```python
from build123d import *

# Parameters (mm, degrees)
SKETCH_W           = 2
SKETCH_H           = 70
PAD_DEPTH          = 25
POLARPATTERN_COUNT = 8
SKETCH001_R        = 70
SKETCH001_R_2      = 67.5
SKETCH001_R_3      = 5
PAD001_DEPTH       = 2


with BuildPart() as part:
    # Sketch → Pad (new body)
    with BuildSketch(Plane.XY):
        with Locations((0, 35)):
            Rectangle(SKETCH_W, SKETCH_H)
    pad = extrude(amount=PAD_DEPTH)

    # PolarPattern: Pad ×8 about axis
    polarpattern_axis = Axis((0, 0, 0), (0, 0, 1))
    for i in range(1, POLARPATTERN_COUNT):
        add(pad.rotate(polarpattern_axis, i * 360 / POLARPATTERN_COUNT))

    # Sketch001 → Pad001 (join)
    with BuildSketch(Plane.XY):
        Circle(SKETCH001_R)
        Circle(SKETCH001_R_2, mode=Mode.SUBTRACT)
        Circle(SKETCH001_R_3)
    extrude(amount=PAD001_DEPTH)


solid = part.part
```
Input: part model. Units: mm. Frame: model coordinates. A direction names the side the tool comes from. Give positions to 0.01 mm unless a question says otherwise; leave off trailing zeros. Order: outer loops, then holes, each group sorted by start corner. A loop starts at its lowest first (then second) coordinate and runs counter-clockwise, first axis right, second up.
1. Set-up query: faces 1 (the face through (64.813, 26.445, 0.986)), 2 (the face through (25.5, -62.5, 1)). Return all of +Z, -Z, +X, -X, +Y, -Y with unobstructed straight access to the full face (end or side cutting, diameter ignored); none if empty.
Computed:
face 1: +Z, -Z, +X, +Y
face 2: +Z, -Z
2. Cut plane D-D (x = -57.5). Return loops of the section in (y, z), and give its area (3 significant figures).
Computed:
outline: (-39.92, 0) - (-35.36, 0) - (-35.36, 2) - (-39.92, 2) - close; (-1, 0) - (1, 0) - (1, 25) - (-1, 25) - close; (35.36, 0) - (39.92, 0) - (39.92, 2) - (35.36, 2) - close
area: 68.3 mm2
3. Cut plane A-A (x = 16). Return loops of the section in (y, z), and give its area (3 significant figures).
Computed:
outline: (-68.15, 0) - (-65.58, 0) - (-65.58, 2) - (-68.15, 2) - close; (-17.41, 0) - (-14.59, 0) - (-14.59, 25) - (-17.41, 25) - close; (-1, 0) - (1, 0) - (1, 25) - (-1, 25) - close; (14.59, 0) - (17.41, 0) - (17.41, 25) - (14.59, 25) - close; (65.58, 0) - (68.15, 0) - (68.15, 2) - (65.58, 2) - close
area: 202 mm2
4. Pin query (flat end, axial travel): pin 1 Ø12.5 at (y, z) = (34, 18) entering from -X; pin 2 Ø10 at (x, z) = (-27.5, 8) entering from -Y; pin 3 Ø17 at (x, y) = (-15, -62.5) entering from +Z; pin 4 Ø8 at (x, y) = (20.5, -12) entering from -Z. Return the tip coordinate at first contact, or that it passes through.
Computed:
pin 1: stops at x = -41.66
pin 2: stops at y = -33.91
pin 3: stops at z = 2
pin 4: passes through
5. Line query: probe 1 along X at (y, z) = (-26.5, 15.75); probe 2 along X at (y, z) = (-15, 19.75); probe 3 along X at (y, z) = (-17.5, 1.75). Output: solid intervals per line, ascending.
Computed:
probe 1: x = -27.91 to -25.09, -1 to 1, 25.09 to 27.91
probe 2: x = -16.41 to -13.59, -1 to 1, 13.59 to 16.41
probe 3: x = -67.78 to -65.19, -18.91 to -16.09, -1 to 1, 16.09 to 18.91, 65.19 to 67.78
6. Cut plane C-C (z = 16.5). Return loops of the section in (x, y).
Computed:
outline: (-70, -1) - (-2.41, -1) - (-50.2, -48.79) - (-48.79, -50.2) - (-1, -2.41) - (-1, -70) - (1, -70) - (1, -2.41) - (48.79, -50.2) - (50.2, -48.79) - (2.41, -1) - (70, -1) - (70, 1) - (2.41, 1) - (50.2, 48.79) - (48.79, 50.2) - (1, 2.41) - (1, 70) - (-1, 70) - (-1, 2.41) - (-48.79, 50.2) - (-50.2, 48.79) - (-2.41, 1) - (-70, 1) - close
7. Cut plane B-B (y = 11.5). Return loops of the section in (x, z).
Computed:
outline: (-69.05, 0) - (-66.51, 0) - (-66.51, 2) - (-69.05, 2) - close; (-12.91, 0) - (-10.09, 0) - (-10.09, 25) - (-12.91, 25) - close; (-1, 0) - (1, 0) - (1, 25) - (-1, 25) - close; (10.09, 0) - (12.91, 0) - (12.91, 25) - (10.09, 25) - close; (66.51, 0) - (69.05, 0) - (69.05, 2) - (66.51, 2) - close
8. Draft query along Y for faces 3 (the face through (-26.445, 64.813, 0.986)), 4 (the face through (25.975, -24.561, 12.325)), 5 (the face through (-26.8, -62.4, 2)). Return one class per face: released by +Y, released by -Y, zero draft, split by the parting line, or undercut.
Computed:
face 3: released by +Y
face 4: undercut
face 5: zero draft
